Model file for the job. Use its own axes, mm. A direction names the side the tool comes from. Round coordinates to 2 decimals unless told otherwise and drop trailing zeros. Loops run counter-clockwise (first coordinate to the right, second up) from the corner with the lowest first, then second, coordinate; pieces in that order, holes last. Notation, with made-up numbers: (86, 69) -> (140, 69) arc R21 ccw to (140, 89) -> close; hole circle Ø11 at (46, 64). An arc over 180 degrees is marked (long way). Use a Markdown table: item, result.
Autodesk Inventor part; units mm, degrees
ref_plane "YZ Plane" through (0, 0, 0) normal (1, 0, 0) x (0, 1, 0)
ref_plane "XZ Plane" through (0, 0, 0) normal (0, 1, 0) x (-1, 0, 0)
ref_plane "XY Plane" through (0, 0, 0) normal (0, 0, 1) x (1, 0, 0)
sketch "Sketch1" plane through (0, 0, 0) normal (0, 1, 0) x (-1, 0, 0)
  line L0 (-75, -75) -> (75, -75)
  line L1 (75, -75) -> (75, 75)
  line L2 (75, 75) -> (-75, 75)
  line L3 (-75, 75) -> (-75, -75)
  line L4 (-75, -75) -> (75, 75) construction
  line L5 (75, -75) -> (-75, 75) construction
  circle A0 centre (0, 0) radius 17.5
  line L6 (65, 65) -> (65, -65) construction
  line L7 (65, -65) -> (-65, -65) construction
  line L8 (-65, -65) -> (-65, 65) construction
  line L9 (-65, 65) -> (65, 65) construction
  line L10 (75, 65) -> (55, 65) construction
  line L11 (55, 65) -> (55, -65) construction
  line L12 (-75, 65) -> (-55, 65) construction
  line L13 (-55, 65) -> (-55, -65) construction
  line L14 (-55, 65) -> (55, 65) construction
  line L15 (-55, 61.43) -> (55, 61.43)
  line L16 (55, 68.57) -> (-55, 68.57)
  arc A1 (-55, 68.57) -> (-55, 61.43) centre (-55, 65) ccw
  arc A2 (55, 61.43) -> (55, 68.57) centre (55, 65) ccw
  line L17 (-55, -65) -> (55, -65) construction
  line L18 (-55, -68.57) -> (55, -68.57)
  line L19 (55, -61.43) -> (-55, -61.43)
  arc A3 (-55, -61.43) -> (-55, -68.57) centre (-55, -65) ccw
  arc A4 (55, -68.57) -> (55, -61.43) centre (55, -65) ccw
  point P0 (0, 65)
  point P1 (0, -65)
  dimension "d0" = 150
  dimension "d1" = 150
  dimension "d2" = 35
  dimension "d3" = 10
  dimension "d4" = 20
  dimension "d5" = 20
  dimension "d6" = 7.14
  dimension "d7" = 7.14
extrude "Extrusion1" add sketch "Sketch1" along normal blind 3
sketch "Sketch2" plane through (0, 3, 0) normal (0, 1, 0) x (1, 0, 0)
  circle A0 centre (0, 0) radius 35 construction
  line L0 (0, 0) -> (35, 0) construction
  line L1 (35, 0) -> (0, 35) construction
  line L2 (0, 35) -> (-35, 0) construction
  line L3 (-35, 0) -> (0, -35) construction
  line L4 (0, -35) -> (35, 0) construction
  dimension "d21" = 70
hole "Hole1" at (0, 3, 35) at (35, 3, 0) at (0, 3, -35) at (-35, 3, 0) direction (0, -1, 0) diameter 5.5 end through all
fillet "Fillet1" radius 8 4 edges at (-75, 1.5, -75) (-75, 1.5, 75) (75, 1.5, 75) (75, 1.5, -75)
properties part number "BaseTopPlate" material "Aluminum"
Q1. Band-saw the part on A-A, the plane x = 0. Give the cut face in (y, z).
Results list:
| item | result |
|---|---|
| outline | (0, -75) -> (3, -75) -> (3, -68.57) -> (0, -68.57) -> close; (0, -61.43) -> (3, -61.43) -> (3, -37.75) -> (0, -37.75) -> close; (0, -32.25) -> (3, -32.25) -> (3, -17.5) -> (0, -17.5) -> close; (0, 17.5) -> (3, 17.5) -> (3, 32.25) -> (0, 32.25) -> close; (0, 37.75) -> (3, 37.75) -> (3, 61.43) -> (0, 61.43) -> close; (0, 68.57) -> (3, 68.57) -> (3, 75) -> (0, 75) -> close |
Q2. Flat gauge pin, fed straight in: pin 1 (5 mm diameter, centred on x = 0, z = -35, fed in from -Y). Where does the tip first touch, or does it go through?
Results list:
| item | result |
|---|---|
| pin 1 | passes through |
Q3. Band-saw the part on C-C, the plane x = -43.5. Give the cut face in (y, z).
Results list:
| item | result |
|---|---|
| outline | (0, -75) -> (3, -75) -> (3, -68.57) -> (0, -68.57) -> close; (0, -61.43) -> (3, -61.43) -> (3, 61.43) -> (0, 61.43) -> close; (0, 68.57) -> (3, 68.57) -> (3, 75) -> (0, 75) -> close |
Q4. Tool access for faces 1 (the face through (58.57, 1.48, -65.08)), 2 (the face through (1, 0, 18)): list every direction of +Z, -Z, +X, -X, +Y, -Y with a clear straight run to the whole face (end or side of a thin tool).
Results list:
| item | result |
|---|---|
| face 1 | +Y, -Y |
| face 2 | +Z, -Z, +X, -X, -Y |
Q5. Band-saw the part on D-D, the plane z = 0. Give the cut face in (x, y), plus the area to 3 significant figures.
Results list:
| item | result |
|---|---|
| outline | (-75, 0) -> (-37.75, 0) -> (-37.75, 3) -> (-75, 3) -> close; (-32.25, 0) -> (-17.5, 0) -> (-17.5, 3) -> (-32.25, 3) -> close; (17.5, 0) -> (32.25, 0) -> (32.25, 3) -> (17.5, 3) -> close; (37.75, 0) -> (75, 0) -> (75, 3) -> (37.75, 3) -> close |
| area | 312 mm² |
Q6. Pull direction Z, two halves, no side cores. Call faces 3 (the face through (-72.719, 1.521, 72.594)), 4 (the face through (-58.57, 1.48, -64.92)), 5 (the face through (72.719, 1.521, -72.594)): released by +Z, released by -Z, zero draft, split by the parting line, or undercut.
Results list:
| item | result |
|---|---|
| face 3 | released by +Z |
| face 4 | undercut |
| face 5 | released by -Z |
Q7. Drill centre lines: L1, parallel to Z at x = 0, y = 2.3; L2, parallel to Z at x = -39, y = 0.55; L3, parallel to Z at x = 35, y = 1.8. Where is each one in solid material? Low to high. Write a range as from..to.
Results list:
| item | result |
|---|---|
| L1 | z = -75..-68.57, -61.43..-37.75, -32.25..-17.5, 17.5..32.25, 37.75..61.43, 68.57..75 |
| L2 | z = -75..-68.57, -61.43..61.43, 68.57..75 |
| L3 | z = -75..-68.57, -61.43..-2.75, 2.75..61.43, 68.57..75 |
Q8. Band-saw the part on B-B, the plane z = 35. Give the cut face in (x, y).
Results list:
| item | result |
|---|---|
| outline | (-75, 0) -> (-2.75, 0) -> (-2.75, 3) -> (-75, 3) -> close; (2.75, 0) -> (75, 0) -> (75, 3) -> (2.75, 3) -> close |
